from build123d import *

# Parameters (mm, degrees)
SKETCH1_R               = 11
BOSS_EXTRUDE1_DEPTH     = 13
HOLE1_D                 = 6.35
HOLE1_DEPTH             = 10
CUT_EXTRUDE2_DEPTH      = 21.273134933
CUT_EXTRUDE2_DEPTH_BACK = 0.5
CHAMFER1_SIZE           = 0.5


with BuildPart() as part:
    # Sketch1 → Boss-Extrude1 (new body)
    with BuildSketch(Plane(origin=(0, 0, 0), x_dir=(1, 0, 0), z_dir=(0, 1, 0))):
        with Locations(Location((0, 0, 0), (0, 0, 90))):
            Circle(SKETCH1_R)
    extrude(amount=BOSS_EXTRUDE1_DEPTH)

    # Hole1
    with Locations(Plane(origin=(0, 0, 0), x_dir=(-1, 0, 0), z_dir=(0, -1, 0))):
        with Locations((0, 0)):
            Hole(HOLE1_D / 2, depth=HOLE1_DEPTH)

    # Sketch5 → Cut-Extrude2 (cut, two sides: drawn at the far end of the back side and taken through both)
    with BuildSketch(Plane(origin=(0, 13, 0), x_dir=(1, 0, 0), z_dir=(0, 1, 0)).offset(-CUT_EXTRUDE2_DEPTH_BACK)):
        Polygon((0.5, 70.617246053), (0.5, 10.988630488), (0.5, 6.988630488), (-0.5, 6.988630488), (-0.5, 10.988630488), (-0.5, 70.617246053), (-0.5, 189.874477184), (0.5, 189.874477184), align=None)
    extrude(amount=CUT_EXTRUDE2_DEPTH + CUT_EXTRUDE2_DEPTH_BACK, mode=Mode.SUBTRACT)

    # Chamfer1
    chamfer1_edges = [part.edges().sort_by_distance(p)[0] for p in [
        (0, 13, 11),
    ]]
    chamfer(chamfer1_edges, length=CHAMFER1_SIZE)


solid = part.part
Source: CAD feature listing. Evaluate the final solid. Frame: model axes, mm. A direction names the side the tool comes from. Give positions to 0.01 mm unless a question says otherwise; leave off trailing zeros. Write each loop counter-clockwise with the first axis right and the second up, starting at its lowest first coordinate (ties: lowest second). Pieces come first, ordered by that corner, then holes. Notation, with made-up numbers: (69.25, 89) -> (74.25, 89) arc R11 ccw to (74.25, 95) -> close; hole circle Ø11 at (-20, 89.5). An arc over 180 degrees is marked (long way). Write item = value, one per line.
Q1. Cut plane A-A on z = 0. Return loops of the section in (x, y) (3 decimals), then the cut area to 3 significant figures.
Here are the results:
outline = (-11, 0) -> (-3.175, 0) -> (-3.175, 10) -> (3.175, 10) -> (3.175, 0) -> (11, 0) -> (11, 12.5) -> (10.5, 13) -> (-10.5, 13) -> (-11, 12.5) -> close
area = 222 mm²
Q2. First-contact query: pin 1 (5 mm diameter, centred on x = 4.5, y = 9.5, fed in from +Z); pin 2 (6 mm diameter, centred on y = 9.5, z = 6, fed in from +X); pin 3 (3 mm diameter, centred on x = -3, y = 11.5, fed in from -Z). Flat tips, straight axial feed; report the tip coordinate or a pass-through.
Here are the results:
pin_1 = 10.82
pin_2 = 10.58
pin_3 = -10.9
Q3. Cut plane C-C on y = 5. Return loops of the section in (x, z) (3 decimals), then the cut area to 3 significant figures.
Here are the results:
outline = circle Ø22 at (0, 0); hole circle Ø6.35 at (0, 0)
area = 348 mm²
Q4. Line query: line 1 (Y direction, x = 0, z = -9); line 2 (Y direction, x = 1, z = 2.5); line 3 (Z direction, x = 1.5, y = 7.5). Output: solid intervals per line, ascending. Write a range as from..to.
Here are the results:
line_1 = 0..12.5
line_2 = 10..13
line_3 = -10.9..-2.8, 2.8..10.9
Q5. Mould query, pull axis Z, two halves, no side actions, for faces 1 (the face through (10.74, 6.16, 2.38)), 2 (the face through (-0.69, 5.07, 3.1)), 3 (the face through (0, 12.5, -9)). Classes: +Z half, -Z half, draft (parallel to the pull), parting line (faces both ways), or undercut.
Here are the results:
face_1 = parting line
face_2 = undercut
face_3 = draft
Q6. Cut plane B-B on x = 0. Return loops of the section in (y, z) (3 decimals), then the cut area to 3 significant figures.
Here are the results:
outline = (0, -11) -> (12.5, -11) -> (12.5, -6.989) -> (13, -6.989) -> (13, 10.5) -> (12.5, 11) -> (0, 11) -> (0, 3.175) -> (10, 3.175) -> (10, -3.175) -> (0, -3.175) -> close
area = 220 mm²
Q7. Reachability of faces 4 (the face through (0, 10, 0)), 5 (the face through (2, 0, 3)) from +Z, -Z, +X, -X, +Y, -Y: full face, straight path, thin tool, end or side. Return the list, or none.
Here are the results:
face_4 = -Y
face_5 = +Z, -Z, +X, -X, -Y
